Answer from the drawing. Dimensions are ordinates in mm from the lowest x, y and z of the part. A direction names the side the tool comes from. Round coordinates to 2 decimals unless told otherwise and drop trailing zeros. Write each loop counter-clockwise with the first axis right and the second up, starting at its lowest first coordinate (ties: lowest second). Pieces come first, ordered by that corner, then holes. Notation, with made-up numbers: (26.25, 72.25) - (35.25, 72.25) arc R21 cw to (35.25, 108.25) - close; hole circle Ø3 at (-18.75, -13.75). An arc over 180 degrees is marked (long way). Answer as CSV lines item,"result". Start each with the question number.
1) Consider line 1 along Z through (x, y) = (30, 2) (1 decimal); line 2 along Y through (x, z) = (34, 26.65); line 3 along X through (y, z) = (7, 25.5) (1 decimal). Determine where each line is inside the solid, lowest interval first.
2) Which of the six approach directions +Z, -Z, +X, -X, +Y, -Y give full straight-line access (tool end or side, diameter ignored) to the marked faces 1 and 2?
3) Find section B-B on x = 3. Determine the outline of the cut face in (y, z).
4) Find section A-A on y = 14.26. Determine the outline of the cut face in (x, z).
5) Find section C-C on z = 4.75. Determine the outline of the cut face in (x, y) (1 decimal).
6) Find section D-D on y = 21.26. Determine the outline of the cut face in (x, z).
7) Each of these flat-tipped pins is pushed along its axis until it touches: pin 1 (12.5 mm diameter, centred on x = 18.5, y = 17, fed in from -Z); pin 2 (4 mm diameter, centred on x = 9.5, z = 7, fed in from +Y); pin 3 (1.8 mm diameter, centred on x = 26.25, y = 7.84, fed in from -Z) (3 decimals). Where does it stop, or does it pass through?
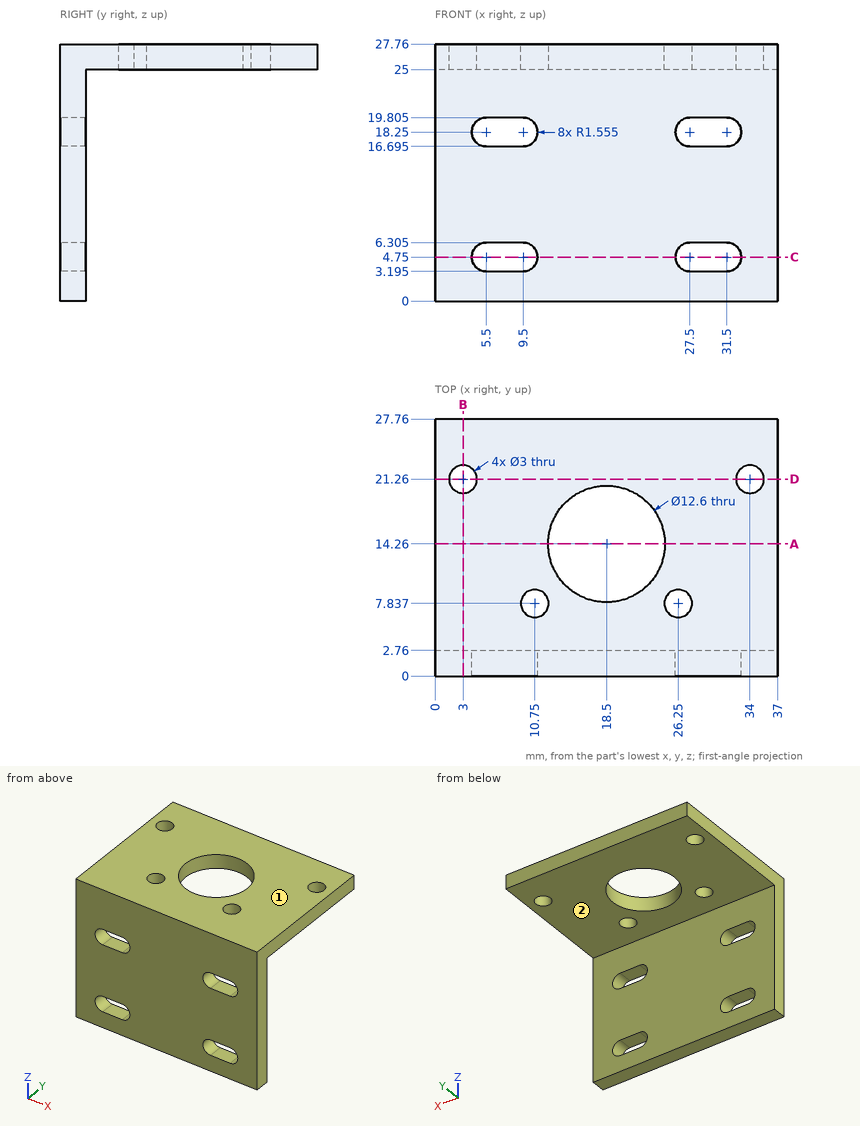
Check values:
1,line 1,"z = 0 to 3.2, 6.3 to 16.7, 19.8 to 27.8"
1,line 2,"y = 0 to 19.76, 22.76 to 27.76"
1,line 3,"x = 0 to 9.5, 12 to 25, 27.5 to 37"
2,face 1,"+Z, +X, -X, +Y, -Y"
2,face 2,"-Z, +X, -X, +Y"
3,outline,"(0, 0) - (2.76, 0) - (2.76, 25) - (19.76, 25) - (19.76, 27.76) - (0, 27.76) - close; (22.76, 25) - (27.76, 25) - (27.76, 27.76) - (22.76, 27.76) - close"
4,outline,"(0, 25) - (12.2, 25) - (12.2, 27.76) - (0, 27.76) - close; (24.8, 25) - (37, 25) - (37, 27.76) - (24.8, 27.76) - close"
5,outline,"(0, 0) - (3.9, 0) - (3.9, 2.8) - (0, 2.8) - close; (11.1, 0) - (25.9, 0) - (25.9, 2.8) - (11.1, 2.8) - close; (33.1, 0) - (37, 0) - (37, 2.8) - (33.1, 2.8) - close"
6,outline,"(0, 25) - (1.5, 25) - (1.5, 27.76) - (0, 27.76) - close; (4.5, 25) - (32.5, 25) - (32.5, 27.76) - (4.5, 27.76) - close; (35.5, 25) - (37, 25) - (37, 27.76) - (35.5, 27.76) - close"
7,pin 1,"stops at z = 25"
7,pin 2,"stops at y = 2.76"
7,pin 3,"passes through"
